```python
from build123d import *

# Parameters (mm, degrees)
F0_W     = 140
F0_H     = 110
F0_W_2   = 134
F0_H_2   = 104
F1_DEPTH = 130
F2_W     = 140
F2_H     = 110
F3_DEPTH = 3


with BuildPart() as f1:
    # F0 (on Top) → F1 (new body)
    with BuildSketch(Plane.XY):
        Rectangle(F0_W, F0_H)
        Rectangle(F0_W_2, F0_H_2, mode=Mode.SUBTRACT)
    extrude(amount=F1_DEPTH)

    # F2 (on Top) → F3 (join)
    with BuildSketch(Plane.XY):
        Rectangle(F2_W, F2_H)
    extrude(amount=-F3_DEPTH)


solid = f1.part
```
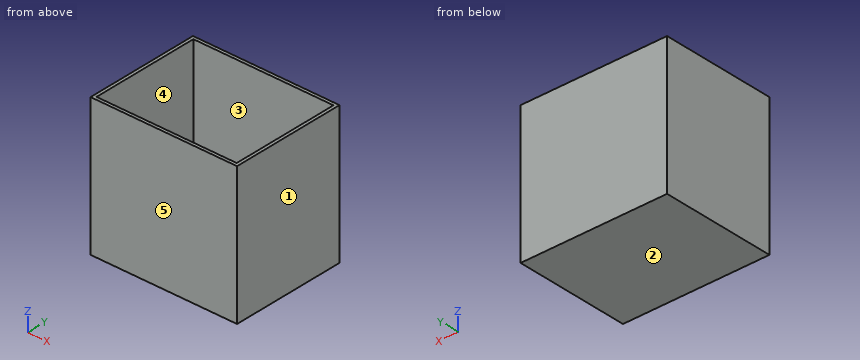
Source: CAD feature listing. Evaluate the final solid. Frame: model axes, mm. Face numbers are marked on the shaded views. A direction names the side the tool comes from. Round coordinates to 2 decimals unless told otherwise and drop trailing zeros. Order: outer loops, then holes, each group sorted by start corner. A loop starts at its lowest first (then second) coordinate and runs counter-clockwise, first axis right, second up. Notation, with made-up numbers: (70.25, 82) -> (77.25, 82) arc R17 cw to (77.25, 98) -> close; hole circle Ø9 at (-16, 26.25). An arc over 180 degrees is marked (long way). One line per item, written item: value. Start each with the question number.
Q1. Section query C-C (x = 6.5). Return the cut outline in (y, z), plus the area to 3 significant figures.
Q2. Section query A-A (z = 12). Return the cut outline in (x, y), plus the area to 3 significant figures.
Q3. Pin query (flat end, axial travel): pin 1 (6 mm diameter, centred on x = -53.5, y = -3, fed in from +Z). Return the tip coordinate at first contact, or that it passes through.
Q4. Section query B-B (y = 27.5). Return the cut outline in (x, z).
Q5. Material intervals for probe 1 along Y at (x, z) = (-25.5, 47); probe 2 along X at (y, z) = (-42, 93); probe 3 along Z at (x, y) = (23.5, -40), sorted ascending.
Q6. Access query for the marked faces 4 and 5. Directions: +Z, -Z, +X, -X, +Y, -Y. A direction counts if a zero-diameter tool reaches every point of the face in a straight line with its end or side. Return the directions, or none.
Q7. Draft query along X for the marked faces 1, 2 and 3. Return one class per face: pulls with the +X half, pulls with the -X half, needs draft (parallel to the pull), parting line crosses it, or undercut.
Findings below:
1. outline: (-55, -3) -> (55, -3) -> (55, 130) -> (52, 130) -> (52, 0) -> (-52, 0) -> (-52, 130) -> (-55, 130) -> close
1. area: 1,110 mm²
2. outline: (-70, -55) -> (70, -55) -> (70, 55) -> (-70, 55) -> close; hole (-67, -52) -> (67, -52) -> (67, 52) -> (-67, 52) -> close
2. area: 1,460 mm²
3. pin 1: z = 0
4. outline: (-70, -3) -> (70, -3) -> (70, 130) -> (67, 130) -> (67, 0) -> (-67, 0) -> (-67, 130) -> (-70, 130) -> close
5. probe 1: -55 to -52, 52 to 55
5. probe 2: -70 to -67, 67 to 70
5. probe 3: -3 to 0
6. face 4: +Z
6. face 5: +Z, -Z, +X, -X, -Y
7. face 1: pulls with the +X half
7. face 2: needs draft
7. face 3: undercut
